CAD build for the part. Positions are in the model's coordinates, mm. A direction names the side the tool comes from. Give positions to 0.01 mm unless a question says otherwise; leave off trailing zeros. Loops run counter-clockwise (first coordinate to the right, second up) from the corner with the lowest first, then second, coordinate; pieces in that order, holes last. Notation, with made-up numbers: M -3.5,79.25 L 10.5,79.25 A6 cw 10.5,88.25 Z; hole C -23.5,30 d5. An arc over 180 degrees is marked long. One line per question, with ' | ' between items.
```python
from build123d import *

# Parameters (mm, degrees)
F0_W     = 197
F0_H     = 145
F1_DEPTH = 20
F2_W     = 6
F2_H     = 20.820669
F2_W_2   = 9.75
F2_H_2   = 7.4


with BuildPart() as f1:
    # F0 (on Top) → F1 (new body)
    with BuildSketch(Plane.XY):
        with Locations((58.305234, 64.482138)):
            Rectangle(F0_W, F0_H)
    extrude(amount=F1_DEPTH)

    # F2 (on face) → F3 (revolve, cut)
    with BuildSketch(Plane.XY.offset(20)):
        with Locations((-26.794766, 4.392473)):
            Rectangle(F2_W, F2_H)
        Polygon((-29.794766, 14.802807), (-23.794766, 14.802807), (-23.794766, 25.102807), (-35.844766, 25.102807), (-40.194766, 25.102807), (-40.194766, 14.802807), align=None)
        Polygon((-35.844766, 25.102807), (-23.794766, 25.102807), (-23.794766, 28.902807), (-33.544766, 28.902807), (-35.844766, 28.902807), align=None)
        with Locations((-28.669766, 32.602807)):
            Rectangle(F2_W_2, F2_H_2)
        Polygon((-29.794766, 40.462807), (-23.794766, 40.462807), (-23.794766, 83.962807), (-33.544766, 83.962807), (-33.544766, 76.562807), (-35.844766, 76.562807), (-35.844766, 72.762807), (-40.194766, 72.762807), (-40.194766, 62.462807), (-29.794766, 62.462807), align=None)
    revolve(axis=Axis((-23.794766, 19.952807, 20), (0, 1, 0)), mode=Mode.SUBTRACT)


solid = f1.part
```
Item 1: Mould opens along Y. For faces 3 (the flat face through (-24, 36.303, 16)), 4 (the cylindrical face through (-23.53, 74.636, 7.953)), 5 (the flat face through (57, 136.982, 10)), 6 (the flat face through (57, -8.018, 10)) say: pulls with the +Y half, pulls with the -Y half, needs draft (parallel to the pull), parting line crosses it, or undercut.
Conclusion:
face 3: undercut | face 4: undercut | face 5: pulls with the +Y half | face 6: pulls with the -Y half
Item 2: Saw through at B-B on z = 18. State how many separate pieces and enclosed holes the cut face has, and give its area (3 significant figures).
Conclusion:
separate pieces: 1 | enclosed holes: 2 | area: 26,900 mm²
Item 3: Saw through at A-A on y = 17. Give the cut face in (x, z), and give its area (3 significant figures).
Conclusion:
outline: M -40.19,0 L 156.81,0 L 156.81,20 L -7.39,20 A16.4 cw -40.19,20 Z | area: 3,520 mm²
Item 4: 3-axis set-ups, long thin cutter, end or side, ignore diameter. For faces 1 (the flat face through (57, 65, 0)), 2 (the cylindrical face through (-23.434, 67.541, 3.604)): which of +Z, -Z, +X, -X, +Y, -Y reach the whole face in a straight line?
Conclusion:
face 1: -Z, +X, -X, +Y, -Y | face 2: +Z
Item 5: Drill centre lines: line 1 along X through (y, z) = (33.5, 12.75); line 2 along X through (y, z) = (78, 15.5); line 3 along Z through (x, y) = (-15, 75). Where is each one in solid material? Low to high. Write a range as [from, to].
Conclusion:
line 1: [-40.19, -30.31], [-17.28, 156.81] | line 2: [-40.19, -32.44], [-15.15, 156.81] | line 3: [0, 11.76]
